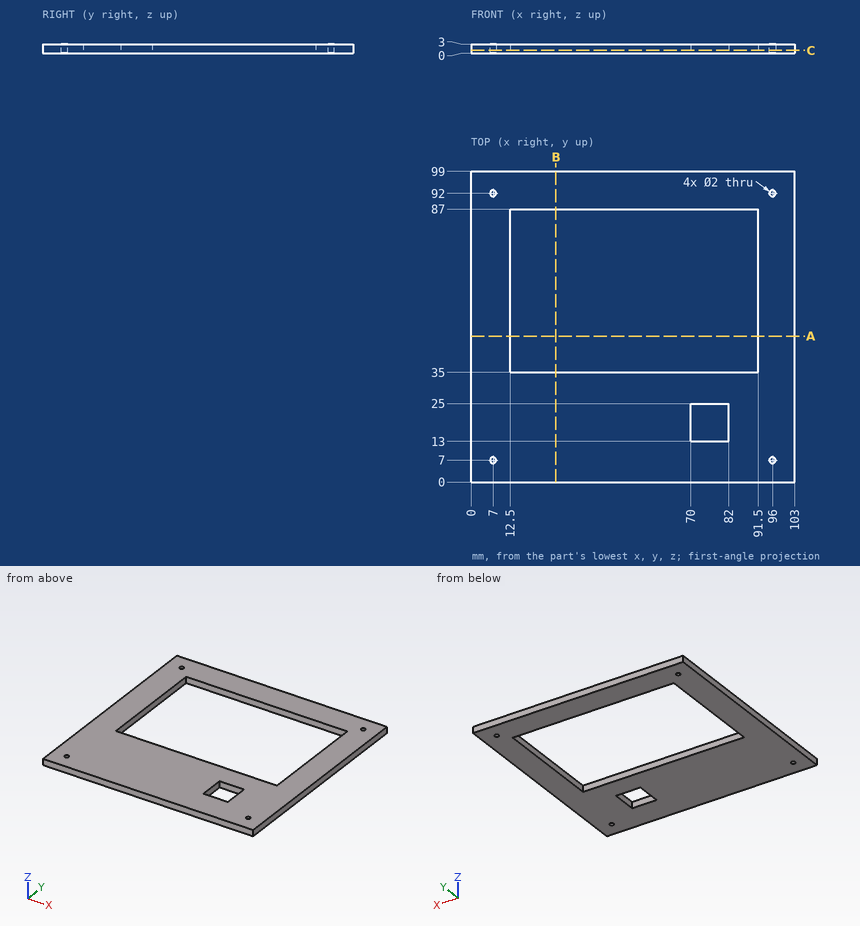
Print and shaded views of the part. All mm, measured from the part's lowest x, y and z. Give positions to 0.01 mm unless a question says otherwise; leave off trailing zeros. Write each loop counter-clockwise with the first axis right and the second up, starting at its lowest first coordinate (ties: lowest second). Pieces come first, ordered by that corner, then holes. Notation, with made-up numbers: (41, 13.25) - (49, 13.25) arc R30 ccw to (49, 36.25) - close; hole circle Ø7 at (48, 44). An arc over 180 degrees is marked (long way). Put each result on its own line as item: value.
(1) Wall check: L1, parallel to Y at x = 96, z = 1.6; L2, parallel to X at y = 92, z = 1.8; L3, parallel to X at y = 83.5, z = 1.75. Give the ranges that are in metal, low to high.
Working result:
L1: 0 to 6, 8 to 91, 93 to 99
L2: 0 to 6, 8 to 95, 97 to 103
L3: 0 to 12.5, 91.5 to 103
(2) Saw through at B-B (x = 27). List the corners of the cut face in (y, z).
Working result:
outline: (0, 0) - (35, 0) - (35, 3) - (0, 3) - close; (87, 0) - (99, 0) - (99, 3) - (87, 3) - close
(3) Saw through at C-C (z = 0.95). List the corners of the cut face in (x, y).
Working result:
outline: (0, 0) - (103, 0) - (103, 99) - (0, 99) - close; hole circle Ø2 at (7, 7); hole circle Ø2 at (7, 92); hole (12.5, 35) - (91.5, 35) - (91.5, 87) - (12.5, 87) - close; hole (70, 13) - (82, 13) - (82, 25) - (70, 25) - close; hole circle Ø2 at (96, 7); hole circle Ø2 at (96, 92)
(4) Saw through at A-A (y = 46.5). List the corners of the cut face in (x, z), then the cut area to 3 significant figures.
Working result:
outline: (0, 0) - (12.5, 0) - (12.5, 3) - (0, 3) - close; (91.5, 0) - (103, 0) - (103, 3) - (91.5, 3) - close
area: 72.0 mm^2
